For this review, use the dimensioned drawing (mm, ordinates from the lowest corner) and the shaded views. Give positions to 0.01 mm unless a question says otherwise; leave off trailing zeros. Write each loop counter-clockwise with the first axis right and the second up, starting at its lowest first coordinate (ties: lowest second). Pieces come first, ordered by that corner, then holes. Notation, with made-up numbers: M -21,-23 L 14,-23 A34 ccw 14,7 Z; hole C -23,54 d2. An arc over 180 degrees is marked long. One line per item, written item: value. Start each with the question number.
Item 1: Consider section C-C, the plane z = 10.75. Write out the cut boundary in (x, y).
Item 2: Consider section A-A, the plane y = 44.45. Write out the cut boundary in (x, z).
Item 3: Mouldability with a two-part tool opening along Y and no side actions: class the marked faces 1, 2 and 3 as released by +Y, released by -Y, zero draft, split by the parting line, or undercut.
Item 4: To check wall thickness, follow probe 1 along Y at (x, z) = (73.5, 10); probe 2 along X at (y, z) = (12, 8) (1 decimal); probe 3 along X at (y, z) = (11.5, 4.5) (1 decimal). State the ranges of each line that lie inside material, in increasing order.
Item 5: Consider section B-B, the plane y = 10. Write out the cut boundary in (x, z).
Item 6: Consider section D-D, the plane x = 63.5. Write out the cut boundary in (y, z), and give its area (3 significant figures).
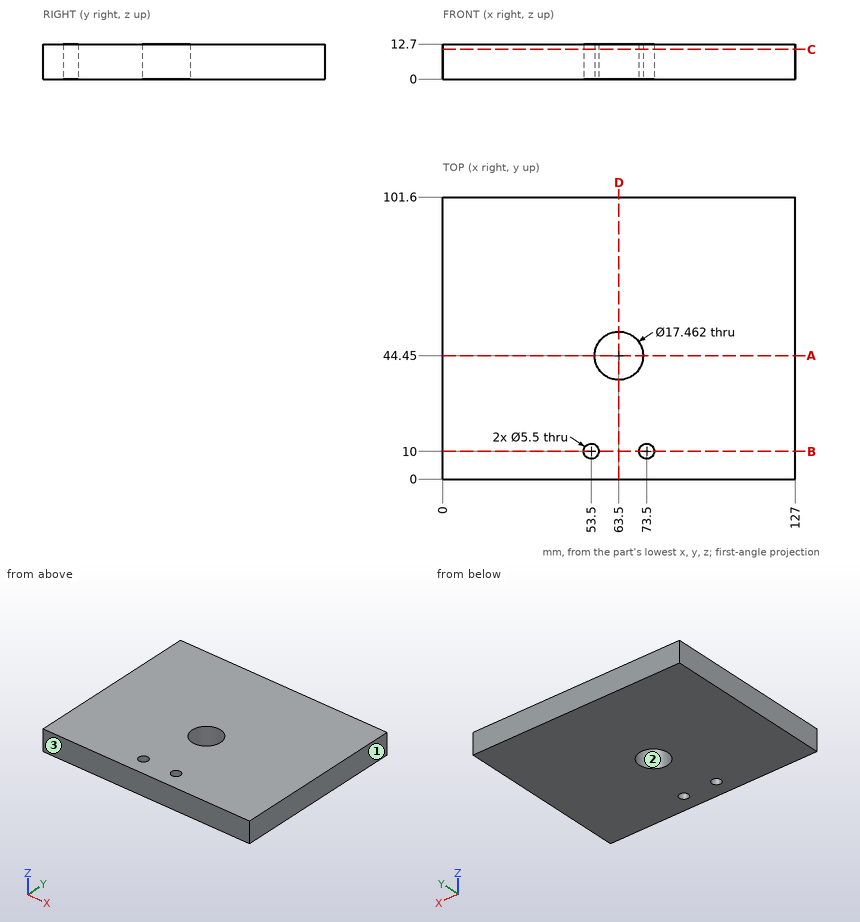
Model answer:
1. outline: M 0,0 L 127,0 L 127,101.6 L 0,101.6 Z; hole C 53.5,10 d5.5; hole C 63.5,44.45 d17.46; hole C 73.5,10 d5.5
2. outline: M 0,0 L 54.77,0 L 54.77,12.7 L 0,12.7 Z; M 72.23,0 L 127,0 L 127,12.7 L 72.23,12.7 Z
3. face 1: zero draft
3. face 2: undercut
3. face 3: released by -Y
4. probe 1: y = 0 to 7.25, 12.75 to 101.6
4. probe 2: x = 0 to 51.6, 55.4 to 71.6, 75.4 to 127
4. probe 3: x = 0 to 51.2, 55.8 to 71.2, 75.8 to 127
5. outline: M 0,0 L 50.75,0 L 50.75,12.7 L 0,12.7 Z; M 56.25,0 L 70.75,0 L 70.75,12.7 L 56.25,12.7 Z; M 76.25,0 L 127,0 L 127,12.7 L 76.25,12.7 Z
6. outline: M 0,0 L 35.72,0 L 35.72,12.7 L 0,12.7 Z; M 53.18,0 L 101.6,0 L 101.6,12.7 L 53.18,12.7 Z
6. area: 1,070 mm2
